Verification items for the finished model (mm, model axes). Face numbers are marked on the shaded views. Round coordinates to 2 decimals unless told otherwise and drop trailing zeros. Loops run counter-clockwise (first coordinate to the right, second up) from the corner with the lowest first, then second, coordinate; pieces in that order, holes last. Notation, with made-up numbers: (41, -22) -> (47, -22) arc R13 cw to (47, -5) -> close; hole circle Ø10 at (46, -2). An arc over 180 degrees is marked (long way). Use a Markdown table: item, result. Add a question column.
```python
from build123d import *

# Parameters (mm, degrees)
F0_R     = 18.415
F0_R_2   = 15.875
F1_DEPTH = 76.2
F2_R     = 10.054491
F3_DEPTH = 40.64
F5_R     = 17.4625
F6_DEPTH = 25.4


with BuildPart() as f1:
    # F0 (on Front) → F1 (new body, symmetric)
    with BuildSketch(Plane.XZ):
        Circle(F0_R)
        Circle(F0_R_2, mode=Mode.SUBTRACT)
    extrude(amount=F1_DEPTH, both=True)

    # F2 (on Top) → F3 (cut, symmetric)
    with BuildSketch(Plane.XY):
        Circle(F2_R)
    extrude(amount=F3_DEPTH, both=True, mode=Mode.SUBTRACT)

    # F5 (on face) → F6 (cut)
    with BuildSketch(Plane.XZ.offset(76.2)):
        Circle(F5_R)
    extrude(amount=-F6_DEPTH, mode=Mode.SUBTRACT)


solid = f1.part
```
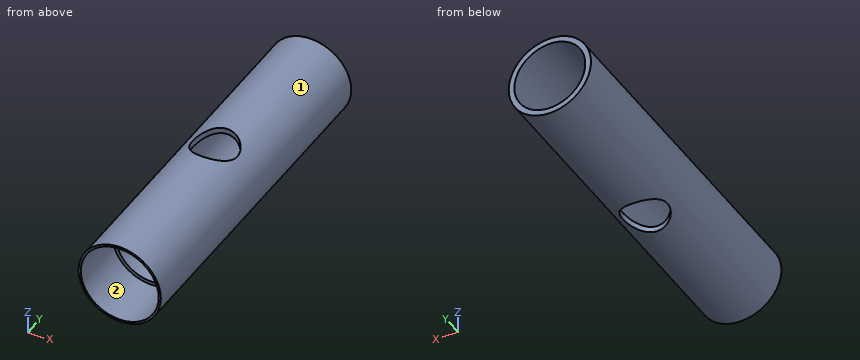
1) Sectioned sample at C-C on x = -12. Enter the section's corners in (y, z), then the cut area to 3 significant figures.
2) Go/stop test with flat-tipped pins: pin 1 (4 mm diameter, centred on y = -14, z = 12.5, fed in from -X); pin 2 (12 mm diameter, centred on x = -11, y = 24.5, fed in from -Z); pin 3 (4 mm diameter, centred on y = -23, z = 13, fed in from -X). Record where each tip stops, or that it passes through.
3) Thickness scan on line 1 (Z direction, x = 0, y = -23.5) (3 decimals); line 2 (Z direction, x = -0.5, y = -56.5); line 3 (Y direction, x = 0, z = 17). Record the ranges inside material, lowest first.
4) Release check for a two-part mould opening along Z. For the marked faces 1 and 2 record: released by +Z, released by -Z, zero draft, split by the parting line, or undercut.
5) Sectioned sample at D-D on y = 24. Enter the section's corners in (x, z) (3 decimals), then the cut area to 3 significant figures.
6) Sectioned sample at A-A on z = 0. Enter the section's corners in (x, y) (1 decimal).
7) Sectioned sample at B-B on x = 2.5. Enter the section's corners in (y, z), then the cut area to 3 significant figures.
Geometry results:
| question | item | result |
|---|---|---|
| 1 | outline | (-76.2, -13.97) -> (76.2, -13.97) -> (76.2, -10.39) -> (-50.8, -10.39) -> (-50.8, -12.69) -> (-76.2, -12.69) -> close; (-76.2, 12.69) -> (-50.8, 12.69) -> (-50.8, 10.39) -> (76.2, 10.39) -> (76.2, 13.97) -> (-76.2, 13.97) -> close |
| 1 | area | 973 mm^2 |
| 2 | pin 1 | x = -15.13 |
| 2 | pin 2 | z = -17.72 |
| 2 | pin 3 | x = -14.77 |
| 3 | line 1 | -18.415 to -15.875, 15.875 to 18.415 |
| 3 | line 2 | -18.41 to -17.46, 17.46 to 18.41 |
| 3 | line 3 | -50.8 to -10.05, 10.05 to 76.2 |
| 4 | face 1 | split by the parting line |
| 4 | face 2 | undercut |
| 5 | outline | circle Ø36.83 at (0, 0); hole circle Ø31.75 at (0, 0) |
| 5 | area | 274 mm^2 |
| 6 | outline | (-18.4, -76.2) -> (-17.5, -76.2) -> (-17.5, -50.8) -> (-15.9, -50.8) -> (-15.9, 76.2) -> (-18.4, 76.2) -> close; (15.9, -50.8) -> (17.5, -50.8) -> (17.5, -76.2) -> (18.4, -76.2) -> (18.4, 76.2) -> (15.9, 76.2) -> close |
| 7 | outline | (-76.2, -18.24) -> (-9.74, -18.24) -> (-9.74, -15.68) -> (-50.8, -15.68) -> (-50.8, -17.28) -> (-76.2, -17.28) -> close; (-76.2, 17.28) -> (-50.8, 17.28) -> (-50.8, 15.68) -> (-9.74, 15.68) -> (-9.74, 18.24) -> (-76.2, 18.24) -> close; (9.74, -18.24) -> (76.2, -18.24) -> (76.2, -15.68) -> (9.74, -15.68) -> close; (9.74, 15.68) -> (76.2, 15.68) -> (76.2, 18.24) -> (9.74, 18.24) -> close |
| 7 | area | 601 mm^2 |
